Check sheet for the modelled part. Datum: model origin and axes. Units: mm. Face numbers are marked on the shaded views. Round coordinates to 2 decimals unless told otherwise and drop trailing zeros. Order: outer loops, then holes, each group sorted by start corner. A loop starts at its lowest first (then second) coordinate and runs counter-clockwise, first axis right, second up.
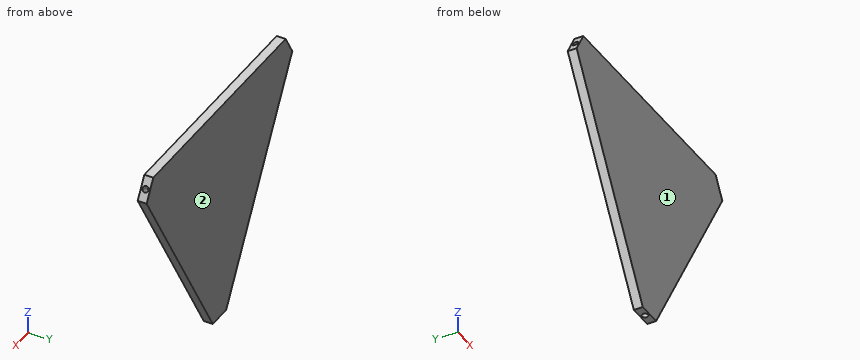
```python
from build123d import *

# Parameters (mm, degrees)
BOSS_EXTRUDE1_DEPTH = 4.7625
CIRPATTERN1_COUNT   = 3


with BuildPart() as part:
    # Sketch1 → Boss-Extrude1 (new, symmetric)
    with BuildSketch(Plane(origin=(0, 0, 0), x_dir=(1, 0, 0), z_dir=(0, 1, 0))):
        Polygon((-12.7, 152.4), (-138.332271537, -65.201477372), (-125.632271537, -87.198522628), (125.632271537, -87.198522628), (138.332271537, -65.201477372), (12.7, 152.4), align=None)
    extrude(amount=BOSS_EXTRUDE1_DEPTH, both=True)

    # Sketch4 → 1/4 (0.25) Diameter Hole1 (revolve, cut)
    with BuildSketch(Plane(origin=(131.982271537, 0, 76.2), x_dir=(0.49999999999999806, 0, -0.8660254037844398), z_dir=(0, 1, 0))):
        Polygon((0, 0), (0, 14.607732465), (3.175, 12.7), (3.175, 0), align=None)
    f_1_4_0_25_diameter_hole1 = revolve(axis=Axis((137.481532851, 0, 79.375), (-0.8660254037844398, 0, -0.49999999999999806)), mode=Mode.SUBTRACT)

    # CirPattern1: 1/4 (0.25) Diameter Hole1 ×3 about axis
    cirpattern1_axis = Axis((0, 4.7625, 0), (0, 1, 0))
    for i in range(1, CIRPATTERN1_COUNT):
        add(f_1_4_0_25_diameter_hole1.rotate(cirpattern1_axis, i * 360 / CIRPATTERN1_COUNT), mode=Mode.SUBTRACT)


solid = part.part
```
Item 1: Sectioned sample at A-A (z = -33). Record the cut outline in (x, y).
Answer:
outline: (-81.64, -4.76) - (81.64, -4.76) - (81.64, 4.76) - (-81.64, 4.76) - close
Item 2: Scan lines: line 1 along Y through (x, z) = (0, -148) (1 decimal); line 2 along X through (y, z) = (0, -146) (3 decimals); line 3 along X through (y, z) = (0, -148) (3 decimals). Record each from-to range of solid material in increasing order.
Answer:
line 1: y = -4.8 to -3.2, 3.2 to 4.8
line 2: x = -16.395 to -3.175, 3.175 to 16.395
line 3: x = -15.24 to -3.175, 3.175 to 15.24
Item 3: Sectioned sample at B-B (x = -33.5). Record the cut outline in (y, z).
Answer:
outline: (-4.76, -116.37) - (4.76, -116.37) - (4.76, 87.2) - (-4.76, 87.2) - close
Item 4: Release check for a two-part mould opening along Y. For the marked faces 1 and 2 record: released by +Y, released by -Y, zero draft, split by the parting line, or undercut.
Answer:
face 1: released by -Y
face 2: released by +Y
Item 5: Go/stop test with flat-tipped pins: P1, Ø1.5, axis at y = 2, z = -29.5, coming from the -X side; P2, Ø3, axis at y = 1, z = 14.5, coming from the +X side; P3, Ø1.5, axis at y = 3, z = 63, coming from the -X side. Record where each tip stops, or that it passes through.
Answer:
P1: stops at x = -84.09
P2: stops at x = 109.93
P3: stops at x = -137.49
